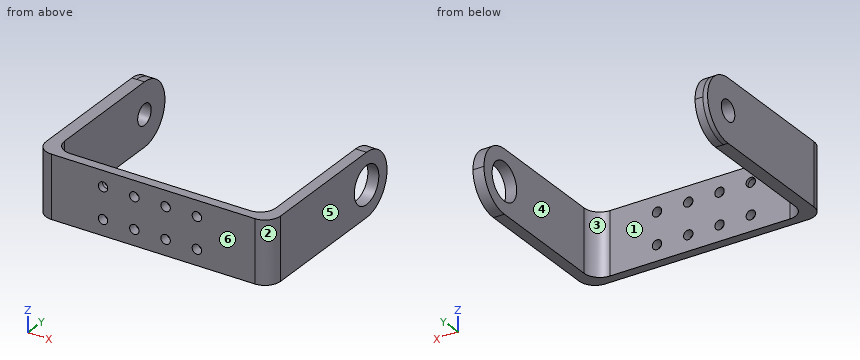
from build123d import *

# Parameters (mm, degrees)
SKETCH_2_R          = 1.5
EXTRUDE_1_DEPTH     = 2
SKETCH_3_W          = 2.5
SKETCH_3_H          = 20
SKETCH_3_W_2        = 3.5
EXTRUDE_2_DEPTH     = 55
SKETCH_9_R          = 6
CUT_EXTRUDE_1_DEPTH = 87
SKETCH_7_R          = 6
SKETCH_7_R_2        = 3.3
EXTRUDE_3_DEPTH     = 2.5
SKETCH_10_R         = 3.3
EXTRUDE_4_DEPTH     = 1.5
SKETCH_11_W         = 67.5
SKETCH_11_H         = 20
SKETCH_11_R         = 1.5
SKETCH_11_R_2       = 1.498871695
EXTRUDE_5_DEPTH     = 1
FILLET_6_R          = 5
FILLET_7_R          = 5
FILLET_8_R          = 5


with BuildPart() as part:
    # 스케치2 → 보스-돌출1 (new body)
    with BuildSketch(Plane(origin=(0, 0, 0), x_dir=(1, 0, 0), z_dir=(0, 1, 0))):
        Polygon((35, -10), (-35, -10), (-35, 10), (35, 10), (38.5, 10), (38.5, -10), align=None)
        with Locations((-15, 5)):
            Circle(SKETCH_2_R, mode=Mode.SUBTRACT)
        with Locations((-5, 5)):
            Circle(SKETCH_2_R, mode=Mode.SUBTRACT)
        with Locations((-15, -5)):
            Circle(SKETCH_2_R, mode=Mode.SUBTRACT)
        with Locations((-5, -5)):
            Circle(SKETCH_2_R, mode=Mode.SUBTRACT)
        with Locations((15, -5)):
            Circle(SKETCH_2_R, mode=Mode.SUBTRACT)
        with Locations((5, -5)):
            Circle(SKETCH_2_R, mode=Mode.SUBTRACT)
        with Locations((5, 5)):
            Circle(SKETCH_2_R, mode=Mode.SUBTRACT)
        with Locations((15, 5)):
            Circle(SKETCH_2_R, mode=Mode.SUBTRACT)
    extrude(amount=EXTRUDE_1_DEPTH)

    # 스케치3 → 보스-돌출2 (add)
    with BuildSketch(Plane(origin=(0, 2, 0), x_dir=(1, 0, 0), z_dir=(0, 1, 0))):
        with Locations((-33.75, 0)):
            Rectangle(SKETCH_3_W, SKETCH_3_H)
        with Locations((36.75, 0)):
            Rectangle(SKETCH_3_W_2, SKETCH_3_H)
    extrude(amount=EXTRUDE_2_DEPTH)

    # 스케치9 → 컷-돌출1 (cut)
    with BuildSketch(Plane(origin=(38.5, 0, 0), x_dir=(0, 0, -1), z_dir=(1, 0, 0))):
        with BuildLine():
            Line((10, 57), (0, 57))
            ThreePointArc((0, 57), (7.071067812, 54.071067812), (10, 47))
            Line((10, 47), (10, 57))
        make_face()
        with BuildLine():
            Line((-10, 57), (-10, 47))
            ThreePointArc((-10, 47), (-7.071067812, 54.071067812), (0, 57))
            Line((0, 57), (-10, 57))
        make_face()
        with Locations((0, 47)):
            Circle(SKETCH_9_R)
    extrude(amount=-CUT_EXTRUDE_1_DEPTH, mode=Mode.SUBTRACT)

    # 스케치7 → 보스-돌출3 (add)
    with BuildSketch(Plane.ZY.offset(35)):
        with Locations((0, 47)):
            Circle(SKETCH_7_R)
        with Locations((0, 47)):
            Circle(SKETCH_7_R_2, mode=Mode.SUBTRACT)
    extrude(amount=-EXTRUDE_3_DEPTH)

    # 스케치10 → 보스-돌출4 (add)
    with BuildSketch(Plane.ZY.offset(35)):
        with BuildLine():
            ThreePointArc((-10, 47), (0, 57), (10, 47))
            Line((10, 47), (10, 0))
            Line((10, 0), (-10, 0))
            Line((-10, 0), (-10, 47))
        make_face()
        with Locations((0, 47)):
            Circle(SKETCH_10_R, mode=Mode.SUBTRACT)
    extrude(amount=EXTRUDE_4_DEPTH)

    # 스케치11 → 보스-돌출5 (add)
    with BuildSketch(Plane(origin=(0, 2, 0), x_dir=(1, 0, 0), z_dir=(0, 1, 0))):
        with Locations((1.25, 0)):
            Rectangle(SKETCH_11_W, SKETCH_11_H)
        with Locations((-15, 5)):
            Circle(SKETCH_11_R, mode=Mode.SUBTRACT)
        with Locations((-5, 5)):
            Circle(SKETCH_11_R, mode=Mode.SUBTRACT)
        with Locations((5, 5)):
            Circle(SKETCH_11_R, mode=Mode.SUBTRACT)
        with Locations((15, 5)):
            Circle(SKETCH_11_R, mode=Mode.SUBTRACT)
        with Locations((15, -5)):
            Circle(SKETCH_11_R, mode=Mode.SUBTRACT)
        with Locations((5, -5)):
            Circle(SKETCH_11_R, mode=Mode.SUBTRACT)
        with Locations((-5, -5)):
            Circle(SKETCH_11_R, mode=Mode.SUBTRACT)
        with Locations((-15, -5)):
            Circle(SKETCH_11_R_2, mode=Mode.SUBTRACT)
    extrude(amount=EXTRUDE_5_DEPTH)

    # 필렛6
    fillet_6_edges = [part.edges().sort_by_distance(p)[0] for p in [
        (-32.5, 3, 0),
    ]]
    fillet(fillet_6_edges, radius=FILLET_6_R)

    # 필렛7
    fillet_7_edges = [part.edges().sort_by_distance(p)[0] for p in [
        (35, 3, 0),
    ]]
    fillet(fillet_7_edges, radius=FILLET_7_R)

    # 필렛8
    fillet_8_edges = [part.edges().sort_by_distance(p)[0] for p in [
        (-36.5, 0, 0),
        (38.5, 0, 0),
    ]]
    fillet(fillet_8_edges, radius=FILLET_8_R)


solid = part.part
For this review, take the finished solid that the model builds, in its own axes (mm). Face numbers are marked on the shaded views. A direction names the side the tool comes from. Round coordinates to 2 decimals unless told otherwise and drop trailing zeros. Loops run counter-clockwise (first coordinate to the right, second up) from the corner with the lowest first, then second, coordinate; pieces in that order, holes last. Notation, with made-up numbers: (-8, 77.25) - (47, 77.25) arc R24 ccw to (47, 105.25) - close; hole circle Ø11 at (-18, 71). An arc over 180 degrees is marked (long way). Use one line per item in the form item = value.
Item 1: Consider section D-D on x = -15. State how many separate pieces and enclosed holes the cut face has, then the cut area to 3 significant figures.
Answers:
separate_pieces = 3
enclosed_holes = 0
area = 42.0 mm^2
Item 2: For line 1 (Z direction, x = -5, y = 1); line 2 (X direction, y = 9, z = -7.25); line 3 (X direction, y = 1, z = -5), list the stretches that pass through material, from the lowest coordinate up.
Answers:
line_1 = -10 to -6.5, -3.5 to 3.5, 6.5 to 10
line_2 = -36.5 to -32.5, 35 to 38.5
line_3 = -34.5 to -16.5, -13.5 to -6.5, -3.5 to 3.5, 6.5 to 13.5, 16.5 to 36.5
Item 3: Consider section B-B on y = 34. Write out the cut boundary in (x, z).
Answers:
outline = (-36.5, -10) - (-32.5, -10) - (-32.5, 10) - (-36.5, 10) - close; (35, -10) - (38.5, -10) - (38.5, 10) - (35, 10) - close
Item 4: Clearance check with flat-ended pins moving along their axes: P1, Ø4, axis at x = 5, z = 5, coming from the +Y side; P2, Ø4, axis at x = -15, z = 5, coming from the -Y side; P3, Ø2.5, axis at x = -15, z = 5, coming from the +Y side. State where each tip first meets the part, or that it passes through.
Answers:
P1 = 3
P2 = 0
P3 = through
Item 5: Tool access review of the marked faces 1 and 2: name each direction out of +Z, -Z, +X, -X, +Y, -Y from which nothing blocks a thin tool from reaching the whole face with its end or side.
Answers:
face_1 = +Z, -Z, +Y
face_2 = +Z, -Z, +X, -Y
Item 6: Mouldability with a two-part tool opening along X and no side actions: class the marked faces 3, 4, 5 and 6 as +X half, -X half, draft (parallel to the pull), parting line (faces both ways), or undercut.
Answers:
face_3 = undercut
face_4 = undercut
face_5 = +X half
face_6 = draft
Item 7: Consider section A-A on x = -5. Write out the cut boundary in (y, z).
Answers:
outline = (0, -10) - (3, -10) - (3, -6.5) - (0, -6.5) - close; (0, -3.5) - (3, -3.5) - (3, 3.5) - (0, 3.5) - close; (0, 6.5) - (3, 6.5) - (3, 10) - (0, 10) - close
Item 8: Consider section C-C on z = -2. Write out the cut boundary in (x, y).
Answers:
outline = (-36.5, 5) arc R5 ccw to (-31.5, 0) - (33.5, 0) arc R5 ccw to (38.5, 5) - (38.5, 41.34) - (35, 41.34) - (35, 8) arc R5 cw to (30, 3) - (-27.5, 3) arc R5 cw to (-32.5, 8) - (-32.5, 44.38) - (-36.5, 44.38) - close; (-36.5, 49.62) - (-32.5, 49.62) - (-32.5, 56.8) - (-36.5, 56.8) - close; (35, 52.66) - (38.5, 52.66) - (38.5, 56.8) - (35, 56.8) - close
